The drawing under review shows one solid part. Ordinate dimensions are in mm from its lowest x, y, z. A direction names the side the tool comes from. Coordinates: 2 decimals unless noted, no trailing zeros. Loops run counter-clockwise (first coordinate to the right, second up) from the corner with the lowest first, then second, coordinate; pieces in that order, holes last. Notation, with made-up numbers: (70.25, 23.5) - (109.25, 23.5) arc R16 ccw to (109.25, 53.5) - close; hole circle Ø1 at (39, -13.5). An arc over 180 degrees is marked (long way). Answer as a JSON object with one key per item and string values. Group by question number.
Item 1: Tool access review of the marked faces 1 and 2: name each direction out of +Z, -Z, +X, -X, +Y, -Y from which nothing blocks a thin tool from reaching the whole face with its end or side.
Item 2: Mouldability with a two-part tool opening along Z and no side actions: class the marked faces 3, 4 and 5 as released by +Z, released by -Z, zero draft, split by the parting line, or undercut.
Item 3: To check wall thickness, follow line 1 (X direction, y = 7, z = 9) (1 decimal); line 2 (X direction, y = 8, z = 6.25); line 3 (X direction, y = 3.25, z = 10.25). State the ranges of each line that lie inside material, in increasing order.
Item 4: We need section B-B (z = 10.5). Give the boundary of the cut face in (x, y).
Item 5: Clearance check with a flat-ended pin moving along its axis: pin 1 (4 mm diameter, centred on x = 11.5, z = 7.5, fed in from +Y). State where the tip first meets the part, or that it passes through.
Item 6: We need section C-C (y = 1.5). State how many separate pieces and enclosed holes the cut face has, then the cut area to 3 significant figures.
Item 7: We need section D-D (x = 41.5). Give the boundary of the cut face in (y, z).
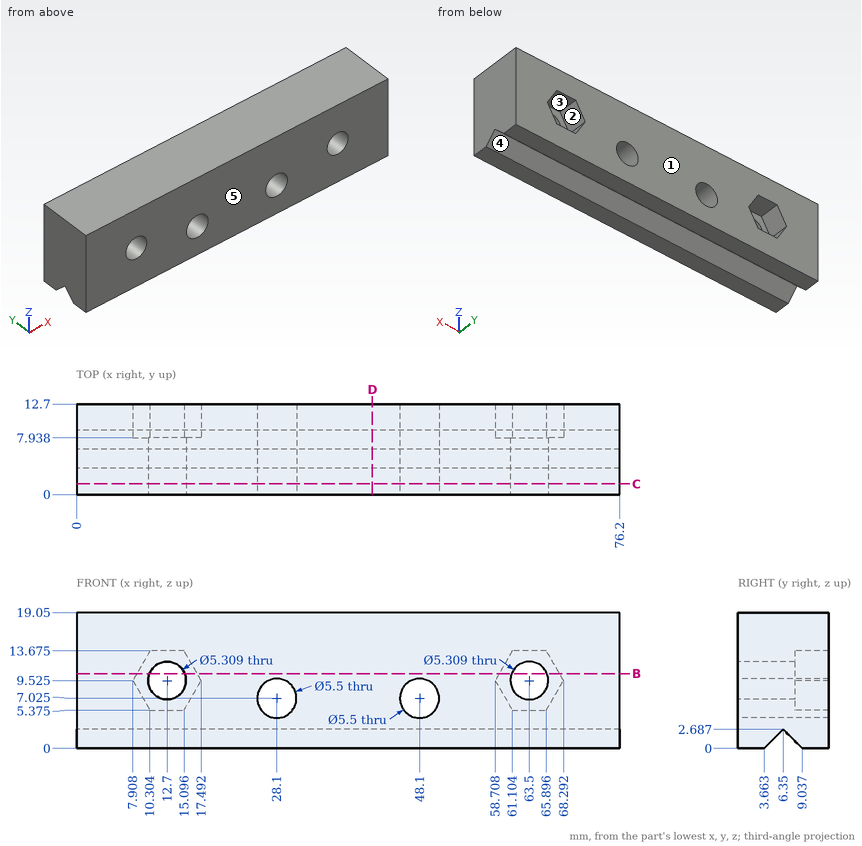
Check sheet entries:
{
 "1": {"face 1": "+Z, -Z, +X, -X, +Y", "face 2": "+Y"},
 "2": {"face 3": "undercut", "face 4": "released by -Z", "face 5": "zero draft"},
 "3": {"line 1": "x = 0 to 10.1, 15.3 to 26.2, 30 to 46.2, 50 to 60.9, 66.1 to 76.2", "line 2": "x = 0 to 9.8, 15.6 to 25.46, 30.74 to 45.46, 50.74 to 60.6, 66.4 to 76.2", "line 3": "x = 0 to 10.15, 15.25 to 60.95, 66.05 to 76.2"},
 "4": {"outline": "(0, 0) - (10.23, 0) - (10.23, 7.94) - (8.47, 7.94) - (8.47, 12.7) - (0, 12.7) - close; (15.17, 0) - (61.03, 0) - (61.03, 7.94) - (59.27, 7.94) - (59.27, 12.7) - (16.93, 12.7) - (16.93, 7.94) - (15.17, 7.94) - close; (65.97, 0) - (76.2, 0) - (76.2, 12.7) - (67.73, 12.7) - (67.73, 7.94) - (65.97, 7.94) - close"},
 "5": {"pin 1": "stops at y = 7.94"},
 "6": {"separate pieces": "1", "enclosed holes": "4", "area": "1,360 mm2"},
 "7": {"outline": "(0, 0) - (3.66, 0) - (6.35, 2.69) - (9.04, 0) - (12.7, 0) - (12.7, 19.05) - (0, 19.05) - close"}
}
